from build123d import *

# Parameters (mm, degrees)
SKETCH_W            = 230
SKETCH_H            = 130
PAD_DEPTH           = 10
SKETCH049_R         = 2.75
HOLE_DEPTH          = 25
PAD024_DEPTH        = 130
HOLE024_D           = 5.5
HOLE024_DEPTH       = 40
HOLE024_CBORE_D     = 14
HOLE024_CBORE_DEPTH = 10
SKETCH050_W         = 65
SKETCH050_H         = 60
POCKET_DEPTH        = 84


with BuildPart() as part:
    # Sketch → Pad (new body)
    with BuildSketch(Plane.XY):
        Rectangle(SKETCH_W, SKETCH_H)
    extrude(amount=PAD_DEPTH)

    # Sketch049 → Hole (cut)
    with BuildSketch(Plane.XY):
        with Locations((-30, 52.5)):
            Circle(SKETCH049_R)
        with Locations((-30, 17.5)):
            Circle(SKETCH049_R)
        with Locations((-30, -17.5)):
            Circle(SKETCH049_R)
        with Locations((-30, -52.5)):
            Circle(SKETCH049_R)
        with Locations((30, -52.5)):
            Circle(SKETCH049_R)
        with Locations((30, -17.5)):
            Circle(SKETCH049_R)
        with Locations((30, 17.5)):
            Circle(SKETCH049_R)
        with Locations((30, 52.5)):
            Circle(SKETCH049_R)
    extrude(amount=HOLE_DEPTH, mode=Mode.SUBTRACT)

    # Sketch051 → Pad024 (join)
    with BuildSketch(Plane.XZ.offset(-65)):
        with BuildLine():
            Line((-105, 30.00001), (-115, 30.00001))
            Line((-115, 30.00001), (-115, 10))
            Line((-115, 10), (-55, 10))
            Line((-55, 10), (-55, 29.999995))
            Line((-55, 29.999995), (-65, 29.999995))
            add(Edge.make_bspline(
                [(-85, 15), (-65.000007, 15), (-65, 29.999995)],
                knots=[4.712389, 4.712389, 4.712389, 6.283185, 6.283185, 6.283185], degree=2, weights=[1, 0.707107, 1]))
            add(Edge.make_bspline(
                [(-105, 30.00001), (-105.000014, 15), (-85, 15)],
                knots=[3.141592, 3.141592, 3.141592, 4.712389, 4.712389, 4.712389], degree=2, weights=[1, 0.707107, 1]))
        make_face()
        with BuildLine():
            Line((65, 30.00001), (55, 30.00001))
            Line((55, 30.00001), (55, 10))
            Line((55, 10), (115, 10))
            Line((115, 10), (115, 29.999995))
            Line((115, 29.999995), (105, 29.999995))
            add(Edge.make_bspline(
                [(85, 15), (104.999993, 15), (105, 29.999995)],
                knots=[4.712389, 4.712389, 4.712389, 6.283185, 6.283185, 6.283185], degree=2, weights=[1, 0.707107, 1]))
            add(Edge.make_bspline(
                [(65, 30.00001), (64.999986, 15), (85, 15)],
                knots=[3.141592, 3.141592, 3.141592, 4.712389, 4.712389, 4.712389], degree=2, weights=[1, 0.707107, 1]))
        make_face()
    extrude(amount=PAD024_DEPTH)

    # Hole024
    with Locations(Plane(origin=(0, 0, 0), x_dir=(1, 0, 0), z_dir=(0, 0, -1))):
        with Locations((-60, 55), (-60, 40), (-110, 55), (-110, 40), (-60, -40), (-60, -55), (-110, -40), (-110, -55), (110, 55), (110, 40), (60, 55), (60, 40), (110, -40), (110, -55), (60, -40), (60, -55)):
            CounterBoreHole(HOLE024_D / 2, HOLE024_CBORE_D / 2, HOLE024_CBORE_DEPTH, depth=HOLE024_DEPTH)

    # Sketch050 → Pocket (cut)
    with BuildSketch(Plane.XY):
        with Locations((-82.5, 0)):
            Rectangle(SKETCH050_W, SKETCH050_H)
        with Locations((82.5, 0)):
            Rectangle(SKETCH050_W, SKETCH050_H)
    extrude(amount=POCKET_DEPTH, mode=Mode.SUBTRACT)


with BuildPart() as part_1:
    # Body placement: moved
    add(part.part.moved(Location((0, 0, 10))))


solid = part_1.part
Verification items for the finished model (mm, model axes). A direction names the side the tool comes from. Give positions to 0.01 mm unless a question says otherwise; leave off trailing zeros. Order: outer loops, then holes, each group sorted by start corner. A loop starts at its lowest first (then second) coordinate and runs counter-clockwise, first axis right, second up. Notation, with made-up numbers: M 32.25,9.5 L 82.25,9.5 A19 cw 82.25,21.5 Z; hole C 24.5,-27.5 d7. An arc over 180 degrees is marked long. Answer as a JSON object with one key per item and string values. Group by question number.
1) Mould release check, pull along X, two halves, no side actions. Record for faces 4 (the face through (-30.358, -49.773, 14.93)), 5 (the face through (115, -48, 28)), 6 (the face through (110, 48, 40)): released by +X, released by -X, zero draft, split by the parting line, or undercut.
2) Access from +Z, -Z, +X, -X, +Y, -Y to the whole of each face (thin tool, end or side, straight path). Record for faces 1 (the face through (29.642, 55.227, 14.93)), 2 (the face through (-106, 40, 20)), 3 (the face through (-1, 1, 20)).
3) Cross-section at A-A (y = -17.5). Enter the section's corners in (x, z), then the cut area to 3 significant figures.
4) Cross-section at C-C (x = 30). Enter the section's corners in (y, z).
5) Cross-section at B-B (z = 31). Give the number of separate pieces and of enclosed holes in the cut face, then the cut area to 3 significant figures.
6) Depth check by flat-ended pin: pin 1 Ø9.5 at (x, y) = (110, 54.5) entering from -Z; pin 2 Ø12 at (x, y) = (-54, -7.5) entering from +Z; pin 3 Ø8 at (y, z) = (-2.5, 15) entering from -X. Enter the tip coordinate at first touch or a pass-through.
7) Scan lines: line 1 along Y through (x, z) = (-60, 24.25); line 2 along Y through (x, z) = (60, 17.5); line 3 along X through (y, z) = (40, 16). Record each from-to range of solid material in increasing order. Write a range as [from, to].
Result sheet:
{
 "1": {"face 4": "undercut", "face 5": "released by +X", "face 6": "zero draft"},
 "2": {"face 1": "+Z, -Z", "face 2": "-Z", "face 3": "+Z, +Y, -Y"},
 "3": {"outline": "M -50,10 L -32.75,10 L -32.75,20 L -50,20 Z; M -27.25,10 L 27.25,10 L 27.25,20 L -27.25,20 Z; M 32.75,10 L 50,10 L 50,20 L 32.75,20 Z", "area": "890 mm2"},
 "4": {"outline": "M -65,10 L -55.25,10 L -55.25,20 L -65,20 Z; M -49.75,10 L -20.25,10 L -20.25,20 L -49.75,20 Z; M -14.75,10 L 14.75,10 L 14.75,20 L -14.75,20 Z; M 20.25,10 L 49.75,10 L 49.75,20 L 20.25,20 Z; M 55.25,10 L 65,10 L 65,20 L 55.25,20 Z"},
 "5": {"separate pieces": "8", "enclosed holes": "16", "area": "3,540 mm2"},
 "6": {"pin 1": "stops at z = 20", "pin 2": "stops at z = 20", "pin 3": "stops at x = -50"},
 "7": {"line 1": "y = [-65, -57.75], [-52.25, -42.75], [-37.25, -30], [30, 37.25], [42.75, 52.25], [57.75, 65]", "line 2": "y = [-65, -62], [-48, -47], [-33, -30], [30, 33], [47, 48], [62, 65]", "line 3": "x = [-103, -67], [-53, 53], [67, 103]"}
}
